```python
from build123d import *

# Parameters (mm, degrees)
SKETCH1_W            = 46.4
SKETCH1_H            = 24.75
BOSS_EXTRUDE1_DEPTH  = 5.9
BOSS_EXTRUDE2_DEPTH  = 2.5
SKETCH3_W            = 50
SKETCH3_H            = 50
BOSS_EXTRUDE3_DEPTH  = 2.5
SKETCH4_W            = 46.4
SKETCH4_H            = 0.93
BOSS_EXTRUDE4_DEPTH  = 5.9
SKETCH5_W            = 46.4
SKETCH5_H            = 0.93
BOSS_EXTRUDE5_DEPTH  = 5.9
SKETCH6_W            = 46.4
SKETCH6_H            = 3
BOSS_EXTRUDE6_DEPTH  = 8.4
SKETCH7_W            = 46.4
SKETCH7_H            = 3
BOSS_EXTRUDE7_DEPTH  = 8.4
SKETCH8_W            = 46.4
SKETCH8_H            = 22.9
BOSS_EXTRUDE8_DEPTH  = 8.4
SKETCH9_W            = 46.4
SKETCH9_H            = 3
BOSS_EXTRUDE9_DEPTH  = 8.4
SKETCH10_W           = 22.9
SKETCH10_H           = 10.9
BOSS_EXTRUDE10_DEPTH = 1.8
SKETCH11_W           = 0.93
SKETCH11_H           = 5.9
BOSS_EXTRUDE11_DEPTH = 1.8
SKETCH12_W           = 32.7
SKETCH12_H           = 0.925
SKETCH12_H_2         = 0.93
BOSS_EXTRUDE12_DEPTH = 8.4
SKETCH13_W           = 0.93
SKETCH13_H           = 5.9
BOSS_EXTRUDE13_DEPTH = 1.8
SKETCH14_W           = 48.2
SKETCH14_H           = 3
BOSS_EXTRUDE14_DEPTH = 8.4
SKETCH15_W           = 32.7
SKETCH15_H           = 0.93
SKETCH15_H_2         = 0.925
BOSS_EXTRUDE15_DEPTH = 8.4
SKETCH16_W           = 0.35
SKETCH16_H           = 5.9
CUT_EXTRUDE1_DEPTH   = 59.371568422
SKETCH18_W           = 0.35
SKETCH18_H           = 5.9
CUT_EXTRUDE2_DEPTH   = 59.371568422
SKETCH20_W           = 22.9
SKETCH20_H           = 2.5
BOSS_EXTRUDE17_DEPTH = 4
SKETCH22_W           = 22.9
SKETCH22_H           = 2.5
BOSS_EXTRUDE19_DEPTH = 3
SKETCH23_W           = 3
SKETCH23_H           = 22.9
BOSS_EXTRUDE20_DEPTH = 1.5
SKETCH24_W           = 22.9
SKETCH24_H           = 2.5
BOSS_EXTRUDE21_DEPTH = 7
SKETCH25_W           = 3
SKETCH25_H           = 22.9
BOSS_EXTRUDE22_DEPTH = 3
SKETCH27_W           = 48.2
SKETCH27_H           = 3
BOSS_EXTRUDE23_DEPTH = 7
SKETCH28_W           = 56.2
SKETCH28_H           = 22.9
BOSS_EXTRUDE24_DEPTH = 7
SKETCH29_W           = 3
SKETCH29_H           = 22.9
BOSS_EXTRUDE25_DEPTH = 7
SKETCH30_W           = 3
SKETCH30_H           = 22.9
BOSS_EXTRUDE26_DEPTH = 7
SKETCH31_W           = 7
SKETCH31_H           = 6.5
CUT_EXTRUDE3_DEPTH   = 56.415182938
SKETCH32_W           = 7
SKETCH32_H           = 6.5
CUT_EXTRUDE4_DEPTH   = 56.415182938
SKETCH33_W           = 2.66
SKETCH33_H           = 2.66
CUT_EXTRUDE5_DEPTH   = 67.259188042
SKETCH34_W           = 2.66
SKETCH34_H           = 2.66
CUT_EXTRUDE6_DEPTH   = 67.259188042
SKETCH35_W           = 3
SKETCH35_H           = 8
CUT_EXTRUDE7_DEPTH   = 3
SKETCH36_W           = 3
SKETCH36_H           = 22.9
BOSS_EXTRUDE27_DEPTH = 1.5
SKETCH38_W           = 48.2
SKETCH38_H           = 3
BOSS_EXTRUDE28_DEPTH = 3.1
SKETCH39_W           = 48.2
SKETCH39_H           = 3
BOSS_EXTRUDE29_DEPTH = 3.1
SKETCH40_W           = 3
SKETCH40_H           = 7.45
BOSS_EXTRUDE30_DEPTH = 0.1
SKETCH41_W           = 3
SKETCH41_H           = 22.9
BOSS_EXTRUDE31_DEPTH = 0.1
SKETCH42_R           = 1
CUT_EXTRUDE8_DEPTH   = 10


with BuildPart() as part:
    # Sketch1 → Boss-Extrude1 (new body)
    with BuildSketch(Plane(origin=(0, 0, 0), x_dir=(1, 0, 0), z_dir=(0, 1, 0))):
        Rectangle(SKETCH1_W, SKETCH1_H)
    extrude(amount=BOSS_EXTRUDE1_DEPTH)

    # Sketch2 → Boss-Extrude2 (add)
    with BuildSketch(Plane(origin=(0, 5.9, 0), x_dir=(1, 0, 0), z_dir=(0, 1, 0))):
        Polygon((23.2, -11.45), (23.2, 0), (23.2, 11.45), (-23.2, 11.45), (-23.2, -11.45), align=None)
    extrude(amount=BOSS_EXTRUDE2_DEPTH)

    # Sketch3 → Boss-Extrude3 (add)
    with BuildSketch(Plane.XZ):
        Rectangle(SKETCH3_W, SKETCH3_H)
    extrude(amount=BOSS_EXTRUDE3_DEPTH)

    # Sketch4 → Boss-Extrude4 (add)
    with BuildSketch(Plane(origin=(0, 0, 0), x_dir=(1, 0, 0), z_dir=(0, 1, 0))):
        with Locations((0, 13.64)):
            Rectangle(SKETCH4_W, SKETCH4_H)
    extrude(amount=BOSS_EXTRUDE4_DEPTH)

    # Sketch5 → Boss-Extrude5 (add)
    with BuildSketch(Plane(origin=(0, 0, 0), x_dir=(1, 0, 0), z_dir=(0, 1, 0))):
        with Locations((0, -13.64)):
            Rectangle(SKETCH5_W, SKETCH5_H)
    extrude(amount=BOSS_EXTRUDE5_DEPTH)

    # Sketch6 → Boss-Extrude6 (add)
    with BuildSketch(Plane(origin=(0, 0, 0), x_dir=(1, 0, 0), z_dir=(0, 1, 0))):
        with Locations((0, 15.605)):
            Rectangle(SKETCH6_W, SKETCH6_H)
    extrude(amount=BOSS_EXTRUDE6_DEPTH)

    # Sketch7 → Boss-Extrude7 (add)
    with BuildSketch(Plane(origin=(0, 0, 0), x_dir=(1, 0, 0), z_dir=(0, 1, 0))):
        with Locations((0, -15.605)):
            Rectangle(SKETCH7_W, SKETCH7_H)
    extrude(amount=BOSS_EXTRUDE7_DEPTH)

    # Sketch8 → Boss-Extrude8 (add)
    with BuildSketch(Plane(origin=(0, 8.4, 0), x_dir=(1, 0, 0), z_dir=(0, 1, 0))):
        Rectangle(SKETCH8_W, SKETCH8_H)
    extrude(amount=BOSS_EXTRUDE8_DEPTH)

    # Sketch9 → Boss-Extrude9 (add)
    with BuildSketch(Plane(origin=(0, 8.4, 0), x_dir=(1, 0, 0), z_dir=(0, 1, 0))):
        with Locations((0, -15.605)):
            Rectangle(SKETCH9_W, SKETCH9_H)
    extrude(amount=BOSS_EXTRUDE9_DEPTH)

    # Sketch10 → Boss-Extrude10 (add)
    with BuildSketch(Plane(origin=(23.2, 0, 0), x_dir=(0, 0, -1), z_dir=(1, 0, 0))):
        with Locations((0, 11.35)):
            Rectangle(SKETCH10_W, SKETCH10_H)
        Polygon((-11.45, 5.9), (11.45, 5.9), (12.375, 5.9), (12.375, 0), (-12.375, 0), (-12.375, 5.9), align=None)
    extrude(amount=BOSS_EXTRUDE10_DEPTH)

    # Sketch11 → Boss-Extrude11 (add)
    with BuildSketch(Plane(origin=(23.2, 0, 0), x_dir=(0, 0, -1), z_dir=(1, 0, 0))):
        Polygon((-14.105, 16.8), (-17.105, 16.8), (-17.105, 0), (-14.105, 0), (-14.105, 5.9), align=None)
        with Locations((-13.64, 2.95)):
            Rectangle(SKETCH11_W, SKETCH11_H)
    extrude(amount=BOSS_EXTRUDE11_DEPTH)

    # Sketch12 → Boss-Extrude12 (add)
    with BuildSketch(Plane(origin=(0, 5.9, 0), x_dir=(1, 0, 0), z_dir=(0, 1, 0))):
        with Locations((-6.85, -11.9125)):
            Rectangle(SKETCH12_W, SKETCH12_H)
        with Locations((-6.85, -13.64)):
            Rectangle(SKETCH12_W, SKETCH12_H_2)
    extrude(amount=BOSS_EXTRUDE12_DEPTH)

    # Sketch13 → Boss-Extrude13 (add)
    with BuildSketch(Plane(origin=(23.2, 0, 0), x_dir=(0, 0, -1), z_dir=(1, 0, 0))):
        Polygon((17.105, 0), (17.105, 8.4), (14.105, 8.4), (14.105, 5.9), (14.105, 0), align=None)
        with Locations((13.64, 2.95)):
            Rectangle(SKETCH13_W, SKETCH13_H)
    extrude(amount=BOSS_EXTRUDE13_DEPTH)

    # Sketch14 → Boss-Extrude14 (add)
    with BuildSketch(Plane(origin=(0, 8.4, 0), x_dir=(1, 0, 0), z_dir=(0, 1, 0))):
        with Locations((0.9, 15.605)):
            Rectangle(SKETCH14_W, SKETCH14_H)
    extrude(amount=BOSS_EXTRUDE14_DEPTH)

    # Sketch15 → Boss-Extrude15 (add)
    with BuildSketch(Plane(origin=(0, 5.9, 0), x_dir=(1, 0, 0), z_dir=(0, 1, 0))):
        with Locations((8.65, 13.64)):
            Rectangle(SKETCH15_W, SKETCH15_H)
        with Locations((8.65, 11.9125)):
            Rectangle(SKETCH15_W, SKETCH15_H_2)
    extrude(amount=BOSS_EXTRUDE15_DEPTH)

    # Sketch16 → Cut-Extrude1 (cut, through all)
    with BuildSketch(Plane(origin=(25, 0, 0), x_dir=(0, 0, -1), z_dir=(1, 0, 0))):
        with Locations((-12.2, 2.95)):
            Rectangle(SKETCH16_W, SKETCH16_H)
        with Locations((-13.35, 2.95)):
            Rectangle(SKETCH16_W, SKETCH16_H)
    extrude(amount=-CUT_EXTRUDE1_DEPTH, mode=Mode.SUBTRACT)

    # Sketch18 → Cut-Extrude2 (cut, through all)
    with BuildSketch(Plane(origin=(25, 0, 0), x_dir=(0, 0, -1), z_dir=(1, 0, 0))):
        with Locations((12.2, 2.95)):
            Rectangle(SKETCH18_W, SKETCH18_H)
        with Locations((13.35, 2.95)):
            Rectangle(SKETCH18_W, SKETCH18_H)
    extrude(amount=-CUT_EXTRUDE2_DEPTH, mode=Mode.SUBTRACT)

    # Sketch20 → Boss-Extrude17 (add)
    with BuildSketch(Plane.ZY.offset(23.2)):
        with Locations((0, 15.55)):
            Rectangle(SKETCH20_W, SKETCH20_H)
    extrude(amount=BOSS_EXTRUDE17_DEPTH)

    # Sketch22 → Boss-Extrude19 (add)
    with BuildSketch(Plane.ZY.offset(27.2)):
        with Locations((0, 15.55)):
            Rectangle(SKETCH22_W, SKETCH22_H)
    extrude(amount=BOSS_EXTRUDE19_DEPTH)

    # Sketch23 → Boss-Extrude20 (add)
    with BuildSketch(Plane(origin=(0, 16.8, 0), x_dir=(1, 0, 0), z_dir=(0, 1, 0))):
        with Locations((-28.7, 0)):
            Rectangle(SKETCH23_W, SKETCH23_H)
    extrude(amount=BOSS_EXTRUDE20_DEPTH)

    # Sketch24 → Boss-Extrude21 (add)
    with BuildSketch(Plane(origin=(25, 0, 0), x_dir=(0, 0, -1), z_dir=(1, 0, 0))):
        with Locations((0, 15.55)):
            Rectangle(SKETCH24_W, SKETCH24_H)
    extrude(amount=BOSS_EXTRUDE21_DEPTH)

    # Sketch25 → Boss-Extrude22 (add)
    with BuildSketch(Plane(origin=(0, 16.8, 0), x_dir=(1, 0, 0), z_dir=(0, 1, 0))):
        with Locations((30.5, 0)):
            Rectangle(SKETCH25_W, SKETCH25_H)
    extrude(amount=BOSS_EXTRUDE22_DEPTH)

    # Sketch27 → Boss-Extrude23 (add)
    with BuildSketch(Plane(origin=(0, 16.8, 0), x_dir=(1, 0, 0), z_dir=(0, 1, 0))):
        with Locations((0.9, 15.605)):
            Rectangle(SKETCH27_W, SKETCH27_H)
        with Locations((0.9, -15.605)):
            Rectangle(SKETCH27_W, SKETCH27_H)
    extrude(amount=BOSS_EXTRUDE23_DEPTH)

    # Sketch28 → Boss-Extrude24 (add)
    with BuildSketch(Plane(origin=(0, 16.8, 0), x_dir=(1, 0, 0), z_dir=(0, 1, 0))):
        with Locations((0.9, 0)):
            Rectangle(SKETCH28_W, SKETCH28_H)
    extrude(amount=BOSS_EXTRUDE24_DEPTH)

    # Sketch29 → Boss-Extrude25 (add)
    with BuildSketch(Plane(origin=(0, 18.3, 0), x_dir=(1, 0, 0), z_dir=(0, 1, 0))):
        with Locations((-28.7, 0)):
            Rectangle(SKETCH29_W, SKETCH29_H)
    extrude(amount=BOSS_EXTRUDE25_DEPTH)

    # Sketch30 → Boss-Extrude26 (add)
    with BuildSketch(Plane(origin=(0, 19.8, 0), x_dir=(1, 0, 0), z_dir=(0, 1, 0))):
        with Locations((30.5, 0)):
            Rectangle(SKETCH30_W, SKETCH30_H)
    extrude(amount=BOSS_EXTRUDE26_DEPTH)

    # Sketch31 → Cut-Extrude3 (cut, through all)
    with BuildSketch(Plane(origin=(0, 0, -11.45), x_dir=(-1, 0, 0), z_dir=(0, 0, -1))):
        with Locations((26.7, 17.55)):
            Rectangle(SKETCH31_W, SKETCH31_H)
    extrude(amount=-CUT_EXTRUDE3_DEPTH, mode=Mode.SUBTRACT)

    # Sketch32 → Cut-Extrude4 (cut, through all)
    with BuildSketch(Plane.XY.offset(11.45)):
        with Locations((28.5, 17.55)):
            Rectangle(SKETCH32_W, SKETCH32_H)
    extrude(amount=-CUT_EXTRUDE4_DEPTH, mode=Mode.SUBTRACT)

    # Sketch33 → Cut-Extrude5 (cut, through all)
    with BuildSketch(Plane.ZY.offset(23.2)):
        with Locations((-12.775, 1.33)):
            Rectangle(SKETCH33_W, SKETCH33_H)
    extrude(amount=-CUT_EXTRUDE5_DEPTH, mode=Mode.SUBTRACT)

    # Sketch34 → Cut-Extrude6 (cut, through all)
    with BuildSketch(Plane.ZY.offset(23.2)):
        with Locations((12.775, 1.33)):
            Rectangle(SKETCH34_W, SKETCH34_H)
    extrude(amount=-CUT_EXTRUDE6_DEPTH, mode=Mode.SUBTRACT)

    # Sketch35 → Cut-Extrude7 (cut)
    with BuildSketch(Plane(origin=(0, 26.8, 0), x_dir=(1, 0, 0), z_dir=(0, 1, 0))):
        with Locations((30.5, 0)):
            Rectangle(SKETCH35_W, SKETCH35_H)
    extrude(amount=-CUT_EXTRUDE7_DEPTH, mode=Mode.SUBTRACT)

    # Sketch36 → Boss-Extrude27 (add)
    with BuildSketch(Plane(origin=(0, 25.3, 0), x_dir=(1, 0, 0), z_dir=(0, 1, 0))):
        with Locations((-28.7, 0)):
            Rectangle(SKETCH36_W, SKETCH36_H)
    extrude(amount=BOSS_EXTRUDE27_DEPTH)

    # Sketch38 → Boss-Extrude28 (add)
    with BuildSketch(Plane(origin=(0, 23.8, 0), x_dir=(1, 0, 0), z_dir=(0, 1, 0))):
        with Locations((0.9, -15.605)):
            Rectangle(SKETCH38_W, SKETCH38_H)
    extrude(amount=BOSS_EXTRUDE28_DEPTH)

    # Sketch39 → Boss-Extrude29 (add)
    with BuildSketch(Plane(origin=(0, 23.8, 0), x_dir=(1, 0, 0), z_dir=(0, 1, 0))):
        with Locations((0.9, 15.605)):
            Rectangle(SKETCH39_W, SKETCH39_H)
    extrude(amount=BOSS_EXTRUDE29_DEPTH)

    # Sketch40 → Boss-Extrude30 (add)
    with BuildSketch(Plane(origin=(0, 26.8, 0), x_dir=(1, 0, 0), z_dir=(0, 1, 0))):
        with Locations((30.5, 7.725)):
            Rectangle(SKETCH40_W, SKETCH40_H)
        with Locations((30.5, -7.725)):
            Rectangle(SKETCH40_W, SKETCH40_H)
    extrude(amount=BOSS_EXTRUDE30_DEPTH)

    # Sketch41 → Boss-Extrude31 (add)
    with BuildSketch(Plane(origin=(0, 26.8, 0), x_dir=(1, 0, 0), z_dir=(0, 1, 0))):
        with Locations((-28.7, 0)):
            Rectangle(SKETCH41_W, SKETCH41_H)
    extrude(amount=BOSS_EXTRUDE31_DEPTH)

    # Sketch42 → Cut-Extrude8 (cut)
    with BuildSketch(Plane(origin=(0, 26.9, 0), x_dir=(1, 0, 0), z_dir=(0, 1, 0))):
        with Locations(Location((-15.7, -15.605, 0), (0, 0, 270))):
            Circle(SKETCH42_R)
        with Locations(Location((-15.7, 15.605, 0), (0, 0, 270))):
            Circle(SKETCH42_R)
        with Locations(Location((17.5, -15.605, 0), (0, 0, 270))):
            Circle(SKETCH42_R)
        with Locations(Location((17.5, 15.605, 0), (0, 0, 270))):
            Circle(SKETCH42_R)
        with Locations(Location((0.9, -15.605, 0), (0, 0, 270))):
            Circle(SKETCH42_R)
        with Locations(Location((0.9, 15.605, 0), (0, 0, 270))):
            Circle(SKETCH42_R)
    extrude(amount=-CUT_EXTRUDE8_DEPTH, mode=Mode.SUBTRACT)


solid = part.part
```
The model under review builds one solid part; all positions refer to its coordinate system, in mm. A direction names the side the tool comes from. Round coordinates to 2 decimals unless told otherwise and drop trailing zeros. Order: outer loops, then holes, each group sorted by start corner. A loop starts at its lowest first (then second) coordinate and runs counter-clockwise, first axis right, second up.
(1) Tool access review of faces 5 (the face through (1, 1, -11.445)), 6 (the face through (29, 25, 8)), 7 (the face through (30, 25, 4)): name each direction out of +Z, -Z, +X, -X, +Y, -Y from which nothing blocks a thin tool from reaching the whole face with its end or side.
Working result:
face 5: +X, -X
face 6: +Z, -Z, +Y
face 7: +X, +Y
(2) Take a section at B-B, the plane z = 9.5. State the section outline as (x, y) points, plus the area to 3 significant figures.
Working result:
outline: (-30.2, 20.8) - (-23.2, 20.8) - (-23.2, 0) - (-25, 0) - (-25, -2.5) - (25, -2.5) - (25, 20.8) - (32, 20.8) - (32, 26.9) - (29, 26.9) - (29, 23.8) - (-27.2, 23.8) - (-27.2, 26.9) - (-30.2, 26.9) - close
area: 1,330 mm2
(3) For P1, Ø18.5, axis at x = 0, z = -0.5, coming from the +Y side; P2, Ø9, axis at x = -6.5, y = 10.5, coming from the +Z side (3 decimals); P3, Ø10, axis at y = 10.5, z = -8, coming from the +X side, all flat-tipped, find the tip position at first contact; note any pin that passes through.
Working result:
P1: stops at y = 23.8
P2: stops at z = 17.105
P3: stops at x = 25
(4) Mouldability with a two-part tool opening along X and no side actions: class faces 1 (the face through (-25, -1, 0)), 2 (the face through (18, 16.9, -16)), 3 (the face through (1, 4, -12.025)), 4 (the face through (32, 23, 0)) as released by +X, released by -X, zero draft, split by the parting line, or undercut.
Working result:
face 1: released by -X
face 2: undercut
face 3: zero draft
face 4: released by +X
(5) Take a section at A-A, the plane y = 19.75. Count the separate pieces of the cut face and the enclosed holes in it, plus the area to 3 significant figures.
Working result:
separate pieces: 3
enclosed holes: 6
area: 1,370 mm2
(6) Take a section at C-C, the plane y = 10. State the section outline as (x, z) points (3 decimals), plus the area to 3 significant figures.
Working result:
outline: (-23.2, -17.105) - (25, -17.105) - (25, -13.175) - (-7.7, -13.175) - (-7.7, -14.105) - (-23.2, -14.105) - close; (-23.2, -11.45) - (-7.7, -11.45) - (-7.7, -12.375) - (25, -12.375) - (25, 11.45) - (9.5, 11.45) - (9.5, 12.375) - (-23.2, 12.375) - close; (-23.2, 13.175) - (9.5, 13.175) - (9.5, 14.105) - (25, 14.105) - (25, 17.105) - (-23.2, 17.105) - close
area: 1,510 mm2
(7) Take a section at D-D, the plane z = -2. State the section outline as (x, y) points.
Working result:
outline: (-30.2, 20.8) - (-23.2, 20.8) - (-23.2, 0) - (-25, 0) - (-25, -2.5) - (25, -2.5) - (25, 20.8) - (32, 20.8) - (32, 23.8) - (-27.2, 23.8) - (-27.2, 26.9) - (-30.2, 26.9) - close
(8) Wall thickness on L1, parallel to Z at x = -19, y = 17.25 (3 decimals); L2, parallel to Z at x = -12, y = 14 (3 decimals); L3, parallel to X at y = 23.25, z = -15: over which ranges is each line inside the solid? List them lowest first.
Working result:
L1: z = -17.105 to -14.105, -11.45 to 11.45, 14.105 to 17.105
L2: z = -17.105 to -14.105, -11.45 to 12.375, 13.175 to 17.105
L3: x = -23.2 to -16.5, -14.9 to 0.1, 1.7 to 16.7, 18.3 to 25
